Could you check a few things on this drawing? It's one solid part, dimensions in mm from its lowest x, y, z. Give positions to 0.01 mm unless a question says otherwise; leave off trailing zeros. Order: outer loops, then holes, each group sorted by start corner. A loop starts at its lowest first (then second) coordinate and runs counter-clockwise, first axis right, second up. Notation, with made-up numbers: M 38,80 L 57,80 A35 ccw 57,119 Z; hole C 15.5,18 d11. An arc over 180 degrees is marked long. Use one line per item in the form item = value.
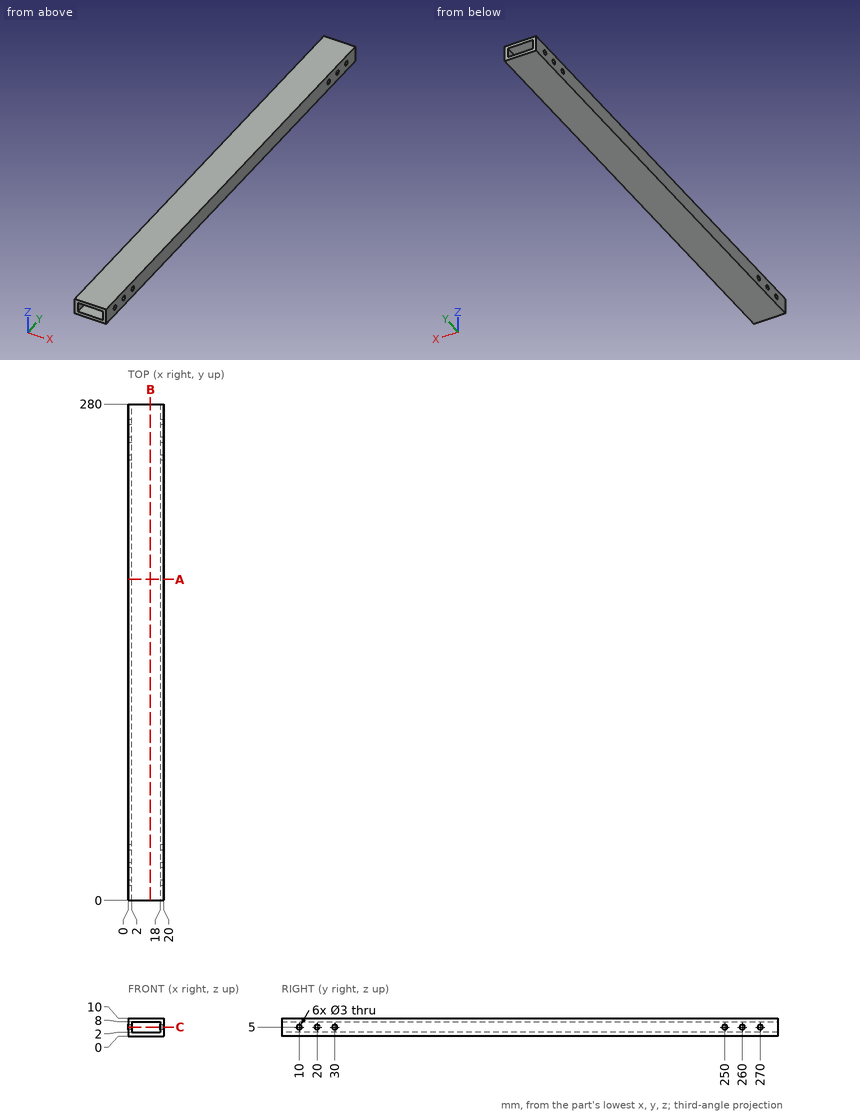
Q1. I want a section at A-A on y = 181. Write out the boundary of the cut face in (x, z), then the cut area to 3 significant figures.
Found:
outline = M 0,0 L 20,0 L 20,10 L 0,10 Z; hole M 2,2 L 18,2 L 18,8 L 2,8 Z
area = 104 mm²
Q2. I'm going to push a flat-ended pin straight in: pin 1 Ø1.8 at (y, z) = (20, 5) entering from +X. Where does the tip first touch, or does it pass through?
Found:
pin_1 = through
Q3. I want a section at C-C on z = 5. State how many separate pieces and enclosed holes the cut face has, then the cut area to 3 significant figures.
Found:
separate_pieces = 14
enclosed_holes = 0
area = 1,050 mm²
Q4. I want a section at B-B on x = 12.5. Write out the boundary of the cut face in (y, z).
Found:
outline = M 0,0 L 280,0 L 280,2 L 0,2 Z; M 0,8 L 280,8 L 280,10 L 0,10 Z
Q5. I need wall thicknesses on L1, parallel to Z at x = 15.25, y = 50; L2, parallel to Z at x = 19.4, y = 260; L3, parallel to X at y = 188.5, z = 7. Which ranges of each line are inside material? Lowest first, please.
Found:
L1 = 0 to 2, 8 to 10
L2 = 0 to 3.5, 6.5 to 10
L3 = 0 to 2, 18 to 20
